from build123d import *

# Parameters (mm, degrees)
BOSS_EXTRUDE1_DEPTH = 4.5


with BuildPart() as part:
    # Model → Boss-Extrude1 (new body)
    with BuildSketch(Plane.XY):
        Polygon((1244.858374133, -975.629345589), (1244.858374133, -1118.40581472), (1156.723196377, -1118.40581472), (1156.723196377, -975.629345589), (1152.29071999, -975.629345589), (1152.29071999, -975.556990867), (1152.29071999, -950.670988096), (1152.29071999, -925.729211157), (1152.29071999, -924.998820047), (1158.083648599, -924.998820047), (1158.083648599, -920.879186992), (1184.295672482, -920.879186992), (1184.295672482, -924.998820047), (1217.264872473, -924.998820047), (1217.264872473, -920.879186992), (1243.476896356, -920.879186992), (1243.476896356, -925.37643338), (1249.290144965, -925.37643338), (1249.290144965, -952.082099206), (1249.290144965, -975.556990867), (1249.290850521, -975.629345589), align=None)
        Polygon((1184.296342759, -971.129347535), (1184.296342759, -975.629345589), (1217.285227751, -975.502557256), (1217.285227751, -971.129347535), align=None, mode=Mode.SUBTRACT)
        with BuildLine():
            add(Edge.make_bspline(
                [(1239.873341912, -1089.255822228), (1239.873341912, -1090.167047227), (1239.134695801, -1090.905693338), (1238.223118024, -1090.905693338), (1237.312245802, -1090.905693338), (1236.572929413, -1090.167047227), (1236.572929413, -1089.255822228)],
                knots=[2, 2, 2, 2, 3, 3, 3, 4, 4, 4, 4], degree=3))
            add(Edge.make_bspline(
                [(1236.572929413, -1089.255822228), (1236.572929413, -1088.344597228), (1237.312245802, -1087.605633617), (1238.223118024, -1087.605633617), (1239.134695801, -1087.605633617), (1239.873341912, -1088.344597228), (1239.873341912, -1089.255822228)],
                knots=[0, 0, 0, 0, 1, 1, 1, 2, 2, 2, 2], degree=3))
        make_face(mode=Mode.SUBTRACT)
        with BuildLine():
            add(Edge.make_bspline(
                [(1165.173317764, -1089.255822228), (1165.173317764, -1090.167047227), (1164.434706931, -1090.905693338), (1163.523129154, -1090.905693338), (1162.612256932, -1090.905693338), (1161.872905265, -1090.167047227), (1161.872905265, -1089.255822228)],
                knots=[2, 2, 2, 2, 3, 3, 3, 4, 4, 4, 4], degree=3))
            add(Edge.make_bspline(
                [(1161.872905265, -1089.255822228), (1161.872905265, -1088.344597228), (1162.612256932, -1087.605633617), (1163.523129154, -1087.605633617), (1164.434706931, -1087.605633617), (1165.173317764, -1088.344597228), (1165.173317764, -1089.255822228)],
                knots=[0, 0, 0, 0, 1, 1, 1, 2, 2, 2, 2], degree=3))
        make_face(mode=Mode.SUBTRACT)
        with BuildLine():
            add(Edge.make_bspline(
                [(1239.873341912, -987.207618087), (1239.873341912, -988.119195864), (1239.134695801, -988.857806697), (1238.223118024, -988.857806697), (1237.312245802, -988.857806697), (1236.572929413, -988.119195864), (1236.572929413, -987.207618087)],
                knots=[2, 2, 2, 2, 3, 3, 3, 4, 4, 4, 4], degree=3))
            add(Edge.make_bspline(
                [(1236.572929413, -987.207618087), (1236.572929413, -986.296745865), (1237.312245802, -985.557746976), (1238.223118024, -985.557746976), (1239.134695801, -985.557746976), (1239.873341912, -986.296745865), (1239.873341912, -987.207618087)],
                knots=[0, 0, 0, 0, 1, 1, 1, 2, 2, 2, 2], degree=3))
        make_face(mode=Mode.SUBTRACT)
        with BuildLine():
            add(Edge.make_bspline(
                [(1165.172964986, -987.207618087), (1165.172964986, -988.119195864), (1164.434354153, -988.857806697), (1163.522776376, -988.857806697), (1162.611904154, -988.857806697), (1161.872587765, -988.119195864), (1161.872587765, -987.207618087)],
                knots=[2, 2, 2, 2, 3, 3, 3, 4, 4, 4, 4], degree=3))
            add(Edge.make_bspline(
                [(1161.872587765, -987.207618087), (1161.872587765, -986.296745865), (1162.611904154, -985.557746976), (1163.522776376, -985.557746976), (1164.434354153, -985.557746976), (1165.172964986, -986.296745865), (1165.172964986, -987.207618087)],
                knots=[0, 0, 0, 0, 1, 1, 1, 2, 2, 2, 2], degree=3))
        make_face(mode=Mode.SUBTRACT)
    extrude(amount=BOSS_EXTRUDE1_DEPTH)


solid = part.part
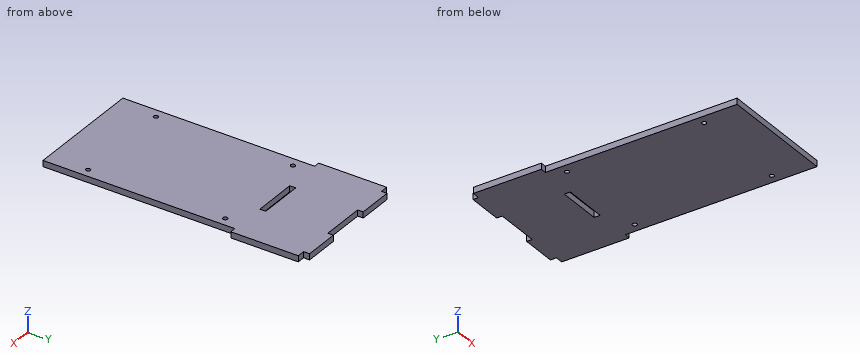
Work out the finished part from the listing and answer in its coordinate system (mm). Round coordinates to 2 decimals unless told otherwise and drop trailing zeros. Loops run counter-clockwise (first coordinate to the right, second up) from the corner with the lowest first, then second, coordinate; pieces in that order, holes last. Notation, with made-up numbers: (-35.75, -5) - (-11.75, -5) arc R37 ccw to (-11.75, 34) - close; hole circle Ø11 at (75, 4.5). An arc over 180 degrees is marked (long way). Use one line per item in the form item = value. Start each with the question number.
(1) Consider line 1 (Y direction, x = 1212, z = 2.7); line 2 (Y direction, x = 1190, z = 0.75); line 3 (X direction, y = -998, z = 1.15). Determine where each line is inside the solid, lowest interval first.
(2) Find section D-D on z = 2.8. Give the number of separate pieces and of enclosed holes in the cut face, and give its area (3 significant figures).
(3) Flat-ended cylindrical pins translate along their axes: P1, Ø1.5, axis at x = 1207, z = 2.5, coming from the +Y side; P2, Ø1.2, axis at y = -923, z = 3.5, coming from the +X side; P3, Ø2, axis at y = -1082.5, z = 3, coming from the +X side. Find the tip coordinate at first contact, or state that the pin passes through.
(4) Find section C-C on y = -1029. Determine the outline of the cut face in (x, z).
(5) Find section A-A on x = 1214. Determine the outline of the cut face in (y, z).
(6) Find section B-B on x = 1190. Determine the outline of the cut face in (y, z), and give its area (3 significant figures).
Answer list:
q1.line_1 = -1118.41 to -975.52, -971.13 to -925
q1.line_2 = -1118.41 to -975.61, -971.13 to -925
q1.line_3 = 1156.72 to 1244.86
q2.separate_pieces = 1
q2.enclosed_holes = 5
q2.area = 17,500 mm^2
q3.P1 = -925
q3.P2 = 1243.48
q3.P3 = 1244.86
q4.outline = (1156.72, 0) - (1244.86, 0) - (1244.86, 4.5) - (1156.72, 4.5) - close
q5.outline = (-1118.41, 0) - (-975.52, 0) - (-975.52, 4.5) - (-1118.41, 4.5) - close; (-971.13, 0) - (-925, 0) - (-925, 4.5) - (-971.13, 4.5) - close
q6.outline = (-1118.41, 0) - (-975.61, 0) - (-975.61, 4.5) - (-1118.41, 4.5) - close; (-971.13, 0) - (-925, 0) - (-925, 4.5) - (-971.13, 4.5) - close
q6.area = 850 mm^2
